from build123d import *

# Parameters (mm, degrees)
SKETCH1_R           = 18.35
SKETCH1_R_2         = 17.2
BOSS_EXTRUDE1_DEPTH = 19
SKETCH1_3_R         = 17.2
BOSS_EXTRUDE2_DEPTH = 30
SKETCH2_R           = 1.5
CUT_EXTRUDE1_DEPTH  = 5
SKETCH2_3_R         = 5.95
SKETCH2_3_R_2       = 2.95
BOSS_EXTRUDE3_DEPTH = 6
SKETCH2_4_R         = 2.95
BOSS_EXTRUDE4_DEPTH = 21
SKETCH3_R           = 13.25
BOSS_EXTRUDE5_DEPTH = 2.9
SKETCH4_R           = 8.85
BOSS_EXTRUDE6_DEPTH = 10.2
SKETCH5_W           = 5.5
SKETCH5_H           = 12.4
BOSS_EXTRUDE7_DEPTH = 6.6
BOSS_EXTRUDE8_DEPTH = 10


with BuildPart() as part:
    # Sketch1 → Boss-Extrude1 (new body)
    with BuildSketch(Plane.XY):
        Circle(SKETCH1_R)
        Circle(SKETCH1_R_2, mode=Mode.SUBTRACT)
        Circle(SKETCH1_R_2)
    extrude(amount=BOSS_EXTRUDE1_DEPTH)

    # Sketch1_3 → Boss-Extrude2 (add)
    with BuildSketch(Plane.XY):
        Circle(SKETCH1_3_R)
    extrude(amount=-BOSS_EXTRUDE2_DEPTH)

    # Sketch2 → Cut-Extrude1 (cut)
    with BuildSketch(Plane.XY.offset(19)):
        with Locations((-7.75, 13.423393759)):
            Circle(SKETCH2_R)
        with Locations((7.75, 13.423393759)):
            Circle(SKETCH2_R)
        with Locations((15.5, 0)):
            Circle(SKETCH2_R)
        with Locations((7.75, -13.423393759)):
            Circle(SKETCH2_R)
        with Locations((-7.75, -13.423393759)):
            Circle(SKETCH2_R)
        with Locations((-15.5, 0)):
            Circle(SKETCH2_R)
    extrude(amount=-CUT_EXTRUDE1_DEPTH, mode=Mode.SUBTRACT)

    # Sketch2_3 → Boss-Extrude3 (add)
    with BuildSketch(Plane.XY.offset(19)):
        with Locations((0, 7.1)):
            Circle(SKETCH2_3_R)
        with Locations((0, 7.1)):
            Circle(SKETCH2_3_R_2, mode=Mode.SUBTRACT)
        with Locations((0, 7.1)):
            Circle(SKETCH2_3_R_2)
    extrude(amount=BOSS_EXTRUDE3_DEPTH)

    # Sketch2_4 → Boss-Extrude4 (add)
    with BuildSketch(Plane.XY.offset(19)):
        with Locations(Location((0, 7.1, 0), (0, 0, 180))):
            Circle(SKETCH2_4_R)
    extrude(amount=BOSS_EXTRUDE4_DEPTH)

    # Sketch3 → Boss-Extrude5 (add)
    with BuildSketch(Plane(origin=(0, 0, -30), x_dir=(-1, 0, 0), z_dir=(0, 0, -1))):
        Circle(SKETCH3_R)
    extrude(amount=BOSS_EXTRUDE5_DEPTH)

    # Sketch4 → Boss-Extrude6 (add)
    with BuildSketch(Plane(origin=(0, 0, -30), x_dir=(-1, 0, 0), z_dir=(0, 0, -1))):
        Circle(SKETCH4_R)
    extrude(amount=BOSS_EXTRUDE6_DEPTH)

    # Sketch5 → Boss-Extrude7 (add)
    with BuildSketch(Plane(origin=(0, 0, -30), x_dir=(-1, 0, 0), z_dir=(0, 0, -1))):
        with Locations((-8.5, 0)):
            Rectangle(SKETCH5_W, SKETCH5_H)
    extrude(amount=BOSS_EXTRUDE7_DEPTH)

    # Sketch6 → Boss-Extrude8 (add)
    with BuildSketch(Plane(origin=(11.25, 0, 0), x_dir=(0, 0, -1), z_dir=(1, 0, 0))):
        with BuildLine():
            ThreePointArc((35.65, 5.071428571), (35.386396103, 5.707824674), (34.75, 5.971428571))
            Line((34.75, 5.971428571), (34.75, 4.171428571))
            ThreePointArc((34.75, 4.171428571), (35.386396103, 4.435032468), (35.65, 5.071428571))
        make_face()
        with BuildLine():
            Line((34.75, 4.171428571), (34.75, 5.971428571))
            ThreePointArc((34.75, 5.971428571), (33.85, 5.071428571), (34.75, 4.171428571))
        make_face()
        with BuildLine():
            ThreePointArc((35.65, 3.042857143), (35.386396103, 3.679253246), (34.75, 3.942857143))
            Line((34.75, 3.942857143), (34.75, 2.142857143))
            ThreePointArc((34.75, 2.142857143), (35.386396103, 2.40646104), (35.65, 3.042857143))
        make_face()
        with BuildLine():
            Line((34.75, 2.142857143), (34.75, 3.942857143))
            ThreePointArc((34.75, 3.942857143), (33.85, 3.042857143), (34.75, 2.142857143))
        make_face()
        with BuildLine():
            ThreePointArc((35.65, 1.014285714), (35.386396103, 1.650681817), (34.75, 1.914285714))
            Line((34.75, 1.914285714), (34.75, 0.114285714))
            ThreePointArc((34.75, 0.114285714), (35.386396103, 0.377889611), (35.65, 1.014285714))
        make_face()
        with BuildLine():
            Line((34.75, 0.114285714), (34.75, 1.914285714))
            ThreePointArc((34.75, 1.914285714), (33.85, 1.014285714), (34.75, 0.114285714))
        make_face()
        with BuildLine():
            ThreePointArc((35.65, -1.014285714), (35.386396103, -0.377889611), (34.75, -0.114285714))
            Line((34.75, -0.114285714), (34.75, -1.914285714))
            ThreePointArc((34.75, -1.914285714), (35.386396103, -1.650681817), (35.65, -1.014285714))
        make_face()
        with BuildLine():
            Line((34.75, -1.914285714), (34.75, -0.114285714))
            ThreePointArc((34.75, -0.114285714), (33.85, -1.014285714), (34.75, -1.914285714))
        make_face()
        with BuildLine():
            ThreePointArc((35.65, -3.042857143), (35.386396103, -2.40646104), (34.75, -2.142857143))
            Line((34.75, -2.142857143), (34.75, -3.942857143))
            ThreePointArc((34.75, -3.942857143), (35.386396103, -3.679253246), (35.65, -3.042857143))
        make_face()
        with BuildLine():
            Line((34.75, -3.942857143), (34.75, -2.142857143))
            ThreePointArc((34.75, -2.142857143), (33.85, -3.042857143), (34.75, -3.942857143))
        make_face()
        with BuildLine():
            ThreePointArc((35.65, -5.071428571), (35.386396103, -4.435032468), (34.75, -4.171428571))
            Line((34.75, -4.171428571), (34.75, -5.971428571))
            ThreePointArc((34.75, -5.971428571), (35.386396103, -5.707824674), (35.65, -5.071428571))
        make_face()
        with BuildLine():
            Line((34.75, -5.971428571), (34.75, -4.171428571))
            ThreePointArc((34.75, -4.171428571), (33.85, -5.071428571), (34.75, -5.971428571))
        make_face()
    extrude(amount=BOSS_EXTRUDE8_DEPTH)


solid = part.part
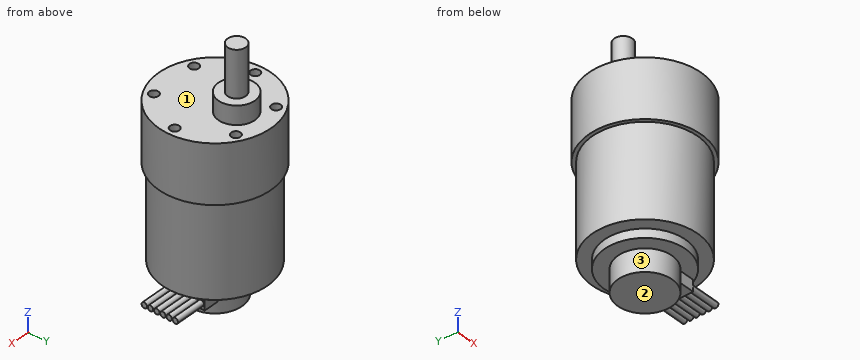
Verification items for the finished model (mm, model axes). Face numbers are marked on the shaded views. Round coordinates to 2 decimals unless told otherwise and drop trailing zeros. Loops run counter-clockwise (first coordinate to the right, second up) from the corner with the lowest first, then second, coordinate; pieces in that order, holes last. Notation, with made-up numbers: (48, 36) - (53, 36) arc R9 ccw to (53, 40) - close; hole circle Ø11 at (59.5, 84). An arc over 180 degrees is marked (long way). Answer in a Markdown table with one row per item. Add a question column.
Q1. Release check for a two-part mould opening along Z. For the marked faces 1, 2 and 3 record: pulls with the +Z half, pulls with the -Z half, needs draft (parallel to the pull), parting line crosses it, or undercut.
Q2. Material ranges on line 1 (Z direction, x = -6.5, y = 14); line 2 (Z direction, x = -6.5, y = 5); line 3 (Y direction, x = -7.75, z = 16.1), recorded low to high.
Q3. Gauge pin test, flat ends, axial feed: pin 1 (2 mm diameter, centred on x = -3, z = 1, fed in from -Y); pin 2 (2 mm diameter, centred on x = 6.5, z = -20, fed in from -Y); pin 3 (1 mm diameter, centred on x = -5.5, y = 5, fed in from +Z). Record the tip position at first contact, or that the pin passes through.
Q4. Section check A-A on x = 15.5. Enter the section's corners in (y, z).
Q5. Section check D-D on z = 20. Enter the section's corners in (x, y), plus the area to 3 significant figures.
Q6. Section check B-B on x = 0. Enter the section's corners in (y, z), plus the area to 3 significant figures.
Q7. Section check C-C on y = 7.1. Enter the section's corners in (x, z), plus the area to 3 significant figures.
Found:
| question | item | result |
|---|---|---|
| 1 | face 1 | pulls with the +Z half |
| 1 | face 2 | pulls with the -Z half |
| 1 | face 3 | needs draft |
| 2 | line 1 | z = -30 to 14 |
| 2 | line 2 | z = -40.2 to 19 |
| 2 | line 3 | y = -16.63 to -14.92, -11.92 to 11.92, 14.92 to 16.63 |
| 3 | pin 1 | stops at y = -18.24 |
| 3 | pin 2 | stops at y = -16.3 |
| 3 | pin 3 | stops at z = 25 |
| 4 | outline | (-9.82, 0) - (-7.46, 0) - (-7.46, -30) - (7.46, -30) - (7.46, 0) - (9.82, 0) - (9.82, 19) - (1.5, 19) - (1.5, 14) - (-1.5, 14) - (-1.5, 19) - (-9.82, 19) - close; circle Ø1.8 at (-5.07, -34.75); circle Ø1.8 at (-3.04, -34.75); circle Ø1.8 at (-1.01, -34.75); circle Ø1.8 at (1.01, -34.75); circle Ø1.8 at (3.04, -34.75); circle Ø1.8 at (5.07, -34.75) |
| 5 | outline | circle Ø11.9 at (0, 7.1) |
| 5 | area | 111 mm² |
| 6 | outline | (-18.35, 0) - (-17.2, 0) - (-17.2, -30) - (-13.25, -30) - (-13.25, -32.9) - (-8.85, -32.9) - (-8.85, -40.2) - (8.85, -40.2) - (8.85, -32.9) - (13.25, -32.9) - (13.25, -30) - (17.2, -30) - (17.2, 0) - (18.35, 0) - (18.35, 19) - (13.05, 19) - (13.05, 25) - (10.05, 25) - (10.05, 40) - (4.15, 40) - (4.15, 25) - (1.15, 25) - (1.15, 19) - (-18.35, 19) - close |
| 6 | area | 2,100 mm² |
| 7 | outline | (-16.92, 0) - (-15.67, 0) - (-15.67, -30) - (-11.19, -30) - (-11.19, -32.9) - (-5.28, -32.9) - (-5.28, -40.2) - (5.28, -40.2) - (5.28, -32.9) - (11.19, -32.9) - (11.19, -30) - (15.67, -30) - (15.67, 0) - (16.92, 0) - (16.92, 19) - (5.95, 19) - (5.95, 25) - (2.95, 25) - (2.95, 40) - (-2.95, 40) - (-2.95, 25) - (-5.95, 25) - (-5.95, 19) - (-16.92, 19) - close |
| 7 | area | 1,880 mm² |
